Verification items for the finished model (mm, model axes). A direction names the side the tool comes from. Coordinates: 2 decimals unless noted, no trailing zeros. Order: outer loops, then holes, each group sorted by start corner. A loop starts at its lowest first (then second) coordinate and runs counter-clockwise, first axis right, second up. Notation, with made-up numbers: M 80.25,15.5 L 98.25,15.5 A22 cw 98.25,25.5 Z; hole C -14,-28 d4. An arc over 180 degrees is marked long. Return JSON: item names as keys, results as strings. Group by question number.
1. Gauge pin test, flat ends, axial feed: pin 1 (1.5 mm diameter, centred on x = -1.5, z = -2.5, fed in from +Y); pin 2 (3 mm diameter, centred on x = 5.5, z = 0, fed in from -Y); pin 3 (1.5 mm diameter, centred on x = -5.5, y = 22.5, fed in from -Z) (3 decimals); pin 4 (6 mm diameter, centred on x = -1.5, z = 4, fed in from +Y). Record the tip position at first contact, or that the pin passes through.
2. Section check C-C, the plane x = -0.75. Record the cut outline in (y, z).
3. Section check A-A, the plane y = 15.75. Record the cut outline in (x, z) (3 decimals).
4. Material ranges on line 1 along Z through (x, y) = (-8.5, 4.75); line 2 along X through (y, z) = (23, 0); line 3 along Z through (x, y) = (-5.25, 19), recorded low to high.
5. Section check B-B, the plane y = 9. Give the number of separate pieces and of enclosed holes in the cut face, plus the area to 3 significant figures.
6. Set-up check for faces 1 (the flat face through (5.475, 24, 2.4)), 2 (the flat face through (4, 7, -0.15)), 3 (the cylindrical face through (-2.865, 21.046, -1.082)): record each of +Z, -Z, +X, -X, +Y, -Y from which the full face is reachable in a straight line by a thin tool's end or side.
7. Mould release check, pull along Z, two halves, no side actions. Record for faces 4 (the flat face through (-10.475, 10, 0)), 5 (the flat face through (-1, 10, 5)), 6 (the cylindrical face through (-10.19, 10.25, -4.7)), 7 (the cylindrical face through (-7.05, 7.826, 1.607)): +Z half, -Z half, draft (parallel to the pull), parting line (faces both ways), or undercut.
Autodesk Inventor part; units mm, degrees
ref_plane "YZ Plane" through (0, 0, 0) normal (1, 0, 0) x (0, 1, 0)
ref_plane "XZ Plane" through (0, 0, 0) normal (0, 1, 0) x (-1, 0, 0)
ref_plane "XY Plane" through (0, 0, 0) normal (0, 0, 1) x (1, 0, 0)
sketch "Skizze5" plane through (0, 0, 0) normal (0, 1, 0) x (-1, 0, 0)
  line L0 (10.475, 5) -> (-10.475, 5) construction
  line L1 (-10.475, 5) -> (-10.475, -5) construction
  line L2 (-10.475, -5) -> (10.475, -5) construction
  line L3 (10.475, -5) -> (10.475, 5) construction
  line L4 (9.475, 5) -> (-7.226, 5)
  line L5 (-7.226, 5) -> (-7.226, -5) construction
  line L6 (-7.226, -5) -> (9.475, -5)
  line L7 (10.475, -4) -> (10.475, 4)
  line L8 (-7.226, -5) -> (-10.475, -2.725)
  line L9 (-10.475, -2.725) -> (-10.475, 2.725)
  line L10 (-7.226, 5) -> (-10.475, 2.725)
  arc A0 (10.475, 4) -> (9.475, 5) centre (9.475, 4) ccw
  arc A1 (9.475, -5) -> (10.475, -4) centre (9.475, -4) ccw
  line L11 (-7.0305, 4.38) -> (9.475, 4.38)
  arc A2 (9.855, 4) -> (9.475, 4.38) centre (9.475, 4) ccw
  line L12 (9.855, 4) -> (9.855, -4)
  arc A3 (9.475, -4.38) -> (9.855, -4) centre (9.475, -4) ccw
  line L13 (9.475, -4.38) -> (-7.0305, -4.38)
  line L14 (-7.0305, -4.38) -> (-9.855, -2.4022)
  line L15 (-9.855, -2.4022) -> (-9.855, 2.4022)
  line L16 (-9.855, 2.4022) -> (-7.0305, 4.38)
  circle A4 centre (5.475, 0) radius 2.25
  circle A5 centre (-5.475, 0) radius 2.25
  line L17 (5.475, 0) -> (-5.475, 0) construction
  point P0 (0, 0)
  point P1 (-10.475, 0)
  point P2 (-10.475, 0)
  point P3 (0, 5)
  point P4 (0, 0)
  dimension "d40" = 20.95
  dimension "d41" = 10
  dimension "d42" = 5.45
  dimension "d43" = 55
  dimension "d44" = 17.701
  dimension "d45" = 1
  dimension "d46" = 0.62
  dimension "d47" = 10.95
  dimension "d48" = 4.5
extrude "Extrusion1" add sketch "Skizze5" along normal blind 14
sketch "Skizze6" plane through (0, 14, 0) normal (0, 1, 0) x (1, 0, 0)
  arc A0 (-9.855, -4) -> (-9.475, -4.38) centre (-9.475, -4) ccw
  line L0 (-9.855, -4) -> (-9.855, 4) construction
  arc A1 (-9.475, 4.38) -> (-9.855, 4) centre (-9.475, 4) ccw construction
  line L1 (-9.475, 4.38) -> (7.0305, 4.38) construction
  line L2 (7.0305, 4.38) -> (9.855, 2.4022) construction
  line L3 (9.855, 2.4022) -> (9.855, -2.4022) construction
  line L4 (9.855, -2.4022) -> (7.0305, -4.38) construction
  line L5 (7.0305, -4.38) -> (-9.475, -4.38) construction
  line L6 (7.226, 5) -> (-9.475, 5)
  arc A2 (-9.475, 5) -> (-10.475, 4) centre (-9.475, 4) ccw
  line L7 (-10.475, 4) -> (-10.475, -4)
  arc A3 (-10.475, -4) -> (-9.475, -5) centre (-9.475, -4) ccw
  line L8 (-9.475, -5) -> (7.226, -5)
  line L9 (7.226, -5) -> (10.475, -2.725)
  line L10 (10.475, -2.725) -> (10.475, 2.725)
  line L11 (10.475, 2.725) -> (7.226, 5)
  point P0 (0, 0)
extrude "Extrusion2" add sketch "Skizze6" along normal blind 6.8
sketch "Skizze7" plane through (-5.475, 0, 0) normal (0, -1, 0) x (1, 0, 0)
  circle A0 centre (0, 0) radius 2.25
  circle A1 centre (10.95, 0) radius 2.25
  point P0 (5.475, 0)
extrude "Extrusion3" cut sketch "Skizze7" against normal blind 1.8
sketch "Skizze8" plane through (0, 20.8, 0) normal (0, 1, 0) x (1, 0, 0)
  circle A0 centre (-5.475, 0) radius 2.25 construction
  circle A1 centre (5.475, 0) radius 2.25 construction
  circle A2 centre (-5.475, 0) radius 2.825
  circle A3 centre (5.475, 0) radius 2.825
  circle A4 centre (-5.475, 0) radius 2.025
  circle A5 centre (5.475, 0) radius 2.025
  point P0 (0, 0)
  dimension "d55" = 5.65
  dimension "d56" = 4.05
extrude "Extrusion4" add sketch "Skizze8" along normal blind 5.5
sketch "Skizze9" plane through (-5.475, 26.3, 0) normal (0, 1, 0) x (1, 0, 0)
  circle A0 centre (0, 0) radius 2.025
  circle A1 centre (0, 0) radius 2.825
  circle A2 centre (10.95, 0) radius 2.025
  circle A3 centre (10.95, 0) radius 2.825
  line L0 (0, 2.825) -> (0, -2.825)
  line L1 (10.95, 2.825) -> (10.95, -2.825)
  point P0 (5.475, 0)
extrude "Extrusion5" cut sketch "Skizze9" against normal blind 4.6 contours L0 A0 | A0 L0 A1 | A2 L1 | A2 L1 A3 picked at (-0.6311, -0.2394) picked at (-2.5397, 0.0814) picked at (11.2429, 0.6082) picked at (13.4678, -0.3597)
sketch "Skizze10" plane through (0, 20.8, 0) normal (0, 1, 0) x (1, 0, 0)
  circle A0 centre (-5.475, 0) radius 2.825
  circle A1 centre (5.475, 0) radius 2.825
  circle A2 centre (-5.475, 0) radius 4.2
  circle A3 centre (5.475, 0) radius 4.2
  circle A4 centre (-5.475, 0) radius 2.025
  circle A5 centre (5.475, 0) radius 2.025
  point P0 (0, 0)
  dimension "d61" = 8.4
extrude "Extrusion6" cut sketch "Skizze10" against normal blind 3
sketch "Skizze11" plane through (-5.475, 1.8, 0) normal (0, -1, 0) x (1, 0, 0)
  circle A0 centre (0, 0) radius 2.25
  circle A1 centre (10.95, 0) radius 2.25
  line L0 (-2.25, 0.15) -> (2.25, 0.15)
  line L1 (2.25, 0.15) -> (2.25, -0.15)
  line L2 (2.25, -0.15) -> (-2.25, -0.15)
  line L3 (-2.25, -0.15) -> (-2.25, 0.15)
  line L4 (-0.15, 2.25) -> (0.15, 2.25)
  line L5 (0.15, 2.25) -> (0.15, -2.25)
  line L6 (0.15, -2.25) -> (-0.15, -2.25)
  line L7 (-0.15, -2.25) -> (-0.15, 2.25)
  line L8 (8.7, 0.15) -> (13.2, 0.15)
  line L9 (13.2, 0.15) -> (13.2, -0.15)
  line L10 (13.2, -0.15) -> (8.7, -0.15)
  line L11 (8.7, -0.15) -> (8.7, 0.15)
  line L12 (10.8, 2.25) -> (11.1, 2.25)
  line L13 (11.1, 2.25) -> (11.1, -2.25)
  line L14 (11.1, -2.25) -> (10.8, -2.25)
  line L15 (10.8, -2.25) -> (10.8, 2.25)
  circle A2 centre (0, 0) radius 1.15
  circle A3 centre (10.95, 0) radius 1.15
  point P0 (5.475, 0)
  point P1 (0, 2.25)
  point P2 (10.95, 2.25)
  point P3 (-2.25, 0)
  point P4 (8.7, 0)
  dimension "d64" = 0.3
  dimension "d68" = 2.3
fillet "Rundung2" radius 0.8 2 edges at (-3.225, 1.8, 0) (7.725, 1.8, 0)
extrude "Extrusion7" cut sketch "Skizze11" against normal up to surface (12.2 mm away) contours A0 L2 A2 L0 | L1 L2 A0 | A0 L0 L1 | L5 A2 L7 A0 | A0 L4 L5 | A2 L2 L5 L0 | L0 L5 A2 | L5 L6 A0 | A0 L7 A2 L5 | A2 L5 L2 | A0 L7 L4 | L5 L0 L7 A2 | L5 L2 L7 L0 | L6 L7 A0 | A2 L7 L2 L5 | L7 L0 A2 | L7 L2 A2 L0 | A2 L2 L7 | L0 A2 L2 A0 | A0 L3 L0 | L2 L3 A0 | A1 L10 A3 L8 | L9 L10 A1 | A1 L8 L9 | L13 A3 L15 A1 | A1 L12 L13 | A3 L10 L13 L8 | L8 L13 A3 | L13 L14 A1 | A1 L15 A3 L13 | A3 L13 L10 | A1 L15 L12 | L13 L8 L15 A3 | L13 L10 L15 L8 | L14 L15 A1 | A3 L15 L10 L13 | L15 L8 A3 | L15 L10 A3 L8 | A3 L10 L15 | L8 A3 L10 A1 | A1 L11 L8 | L10 L11 A1
sketch "Skizze12" plane through (5.475, 17.8, 0) normal (0, 1, 0) x (1, 0, 0)
  circle A0 centre (0, 0) radius 2.025
  circle A1 centre (-10.95, 0) radius 2.025
  point P0 (-5.475, 0)
extrude "Extrusion8" cut sketch "Skizze12" against normal blind 3
chamfer "Fase1" distance 2 angle 45 2 edges at (3.45, 14.8, 0) (-7.5, 14.8, 0)
sketch "Skizze13" plane through (0, 14, 0) normal (0, -1, 0) x (1, 0, 0)
  circle A0 centre (5.475, 0) radius 2.825
  circle A1 centre (-5.475, 0) radius 2.825
  point P0 (0, 0)
extrude "Extrusion9" add sketch "Skizze13" along normal blind 0.8
properties part number "XT90 Male" material "PPS-Kunststoff"
Answers follow:
{
 "1": {"pin 1": "y = 20.8", "pin 2": "y = 1.8", "pin 3": "z = -2.825", "pin 4": "y = 26.3"},
 "2": {"outline": "M 0,-5 L 20.8,-5 L 20.8,5 L 0,5 L 0,4.38 L 14,4.38 L 14,-4.38 L 0,-4.38 Z"},
 "3": {"outline": "M -10.475,-4 A1 ccw -9.475,-5 L 7.226,-5 L 10.475,-2.725 L 10.475,2.725 L 7.226,5 L -9.475,5 A1 ccw -10.475,4 Z; hole C -5.475,0 d1.95; hole C 5.475,0 d1.95"},
 "4": {"line 1": "-5 to -4.38, 4.38 to 5", "line 2": "-3.45 to -2.65, 2.65 to 3.45", "line 3": "-5 to -4.19, -2.82 to -2.01, 2.01 to 2.82, 4.19 to 5"},
 "5": {"separate pieces": "9", "enclosed holes": "1", "area": "55.5 mm^2"},
 "6": {"face 1": "+Z, -Z, +X, +Y", "face 2": "-Y", "face 3": "+Y"},
 "7": {"face 4": "draft", "face 5": "+Z half", "face 6": "-Z half", "face 7": "undercut"}
}
